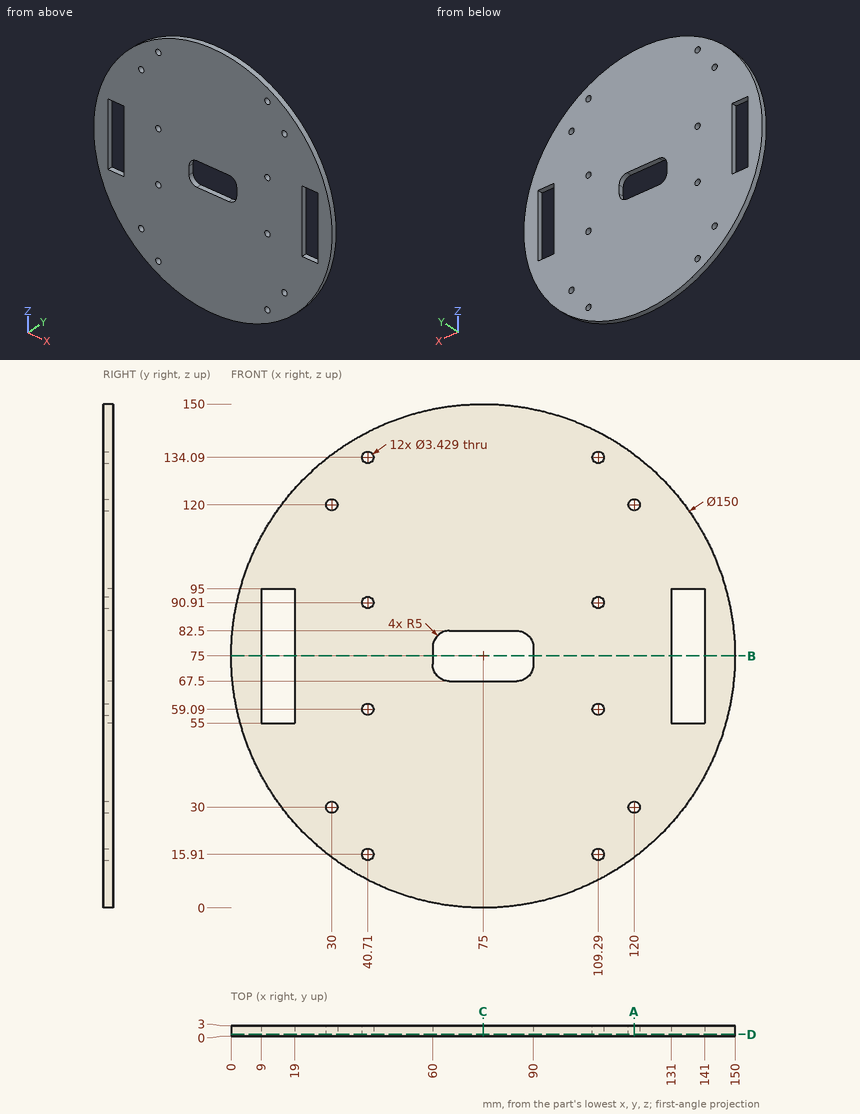
Here's the drawing with two shaded views (mm, measured from the low corner). I have some questions. Round coordinates to 2 decimals unless told otherwise and drop trailing zeros. Loops run counter-clockwise (first coordinate to the right, second up) from the corner with the lowest first, then second, coordinate; pieces in that order, holes last. Notation, with made-up numbers: M 84.25,67 L 97.25,67 A13 cw 97.25,82 Z; hole C 52,55 d10. An arc over 180 degrees is marked long. Answer as a JSON object with one key per item and string values. Group by question number.
Q1. Imagine slicing it at C-C, the plane x = 75. Please give me the cut outline in (y, z).
Q2. Imagine slicing it at D-D, the plane y = 0.5. Count the separate pieces of the cut face and the enclosed holes in it, then the cut area to 3 significant figures.
Q3. Imagine slicing it at B-B, the plane z = 75. Please give me the cut outline in (x, y), then the cut area to 3 significant figures.
Q4. Imagine slicing it at A-A, the plane x = 120. Please give me the cut outline in (y, z).
Q5. Please list where these lines run through material, in increasing order: L1, parallel to Z at x = 28.5, y = 0.75; L2, parallel to X at y = 2.5, z = 135.5; L3, parallel to Z at x = 40.71, y = 0.9.
Q6. Will these pins go through, and if not, where does the flat tip stop? pin 1 (4 mm diameter, centred on x = 109.29, z = 15.91, fed in from -Y); pin 2 (0.9 mm diameter, centred on y = 2, z = 76, fed in from +X); pin 3 (1.5 mm diameter, centred on x = 134, y = 1.5, fed in from -Z); pin 4 (1.5 mm diameter, centred on y = 2.5, z = 115.5, fed in from -X).
Findings:
{
 "1": {"outline": "M 0,0 L 3,0 L 3,67.5 L 0,67.5 Z; M 0,82.5 L 3,82.5 L 3,150 L 0,150 Z"},
 "2": {"separate pieces": "1", "enclosed holes": "15", "area": "16,300 mm2"},
 "3": {"outline": "M 0,0 L 9,0 L 9,3 L 0,3 Z; M 19,0 L 60,0 L 60,3 L 19,3 Z; M 90,0 L 131,0 L 131,3 L 90,3 Z; M 141,0 L 150,0 L 150,3 L 141,3 Z", "area": "300 mm2"},
 "4": {"outline": "M 0,15 L 3,15 L 3,28.29 L 0,28.29 Z; M 0,31.71 L 3,31.71 L 3,118.29 L 0,118.29 Z; M 0,121.71 L 3,121.71 L 3,135 L 0,135 Z"},
 "5": {"L1": "z = 16.15 to 29.17, 30.83 to 119.17, 120.83 to 133.85", "L2": "x = 30.67 to 39.73, 41.69 to 108.31, 110.27 to 119.33", "L3": "z = 8.3 to 14.2, 17.62 to 57.38, 60.8 to 89.2, 92.62 to 132.38, 135.8 to 141.7"},
 "6": {"pin 1": "stops at y = 0", "pin 2": "stops at x = 150", "pin 3": "stops at z = 27.76", "pin 4": "stops at x = 11.4"}
}
